```python
from build123d import *

# Parameters (mm, degrees)
F0_R     = 9.525
F1_DEPTH = 152.4
F2_SIZE2 = 1.27
F2_SIZE  = 1.27
F3_SIZE2 = 1.27
F3_SIZE  = 1.27


with BuildPart() as f1:
    # F0 (on Front) → F1 (new body)
    with BuildSketch(Plane.XZ):
        Circle(F0_R)
    extrude(amount=F1_DEPTH)

    # F2
    f2_edges = [f1.edges().sort_by_distance(p)[0] for p in [
        (-9.525, 0, 0),
    ]]
    chamfer(f2_edges, length=F2_SIZE, length2=F2_SIZE2)

    # F3
    f3_edges = [f1.edges().sort_by_distance(p)[0] for p in [
        (-9.525, -152.4, 0),
    ]]
    chamfer(f3_edges, length=F3_SIZE, length2=F3_SIZE2)


solid = f1.part
```
Build history of the part. All positions in model axes, mm. Round coordinates to 2 decimals unless told otherwise and drop trailing zeros. Loops run counter-clockwise (first coordinate to the right, second up) from the corner with the lowest first, then second, coordinate; pieces in that order, holes last.
Item 1: Pin check, flat tips, straight feed: P1, Ø6, axis at x = 4, y = -39.5, coming from the -Z side; P2, Ø1.5, axis at y = -60.5, z = -5.5, coming from the +X side; P3, Ø1, axis at y = -101, z = 1.5, coming from the +X side. Stop position of each tip, or through.
Item 2: Drill centre lines: line 1 along X through (y, z) = (-109.5, -4.75); line 2 along X through (y, z) = (-29.5, 1); line 3 along Z through (x, y) = (-1.5, -145). Where is each one in solid material? Low to high.
Item 3: Saw through at A-A (y = -92). List the corners of the cut face in (x, z) (3 decimals), then the cut area to 3 significant figures.
Worked answers:
1. P1: stops at z = -9.47
1. P2: stops at x = 8.26
1. P3: stops at x = 9.47
2. line 1: x = -8.26 to 8.26
2. line 2: x = -9.47 to 9.47
2. line 3: z = -9.41 to 9.41
3. outline: circle Ø19.05 at (0, 0)
3. area: 285 mm2
